Print and shaded views of the part. All mm, measured from the part's lowest x, y and z. A direction names the side the tool comes from. Coordinates: 2 decimals unless noted, no trailing zeros. Order: outer loops, then holes, each group sorted by start corner. A loop starts at its lowest first (then second) coordinate and runs counter-clockwise, first axis right, second up. Notation, with made-up numbers: M 34.25,73.5 L 60.25,73.5 A20 cw 60.25,94.5 Z; hole C 70,2 d8. An arc over 180 degrees is marked long. One line per item, written item: value.
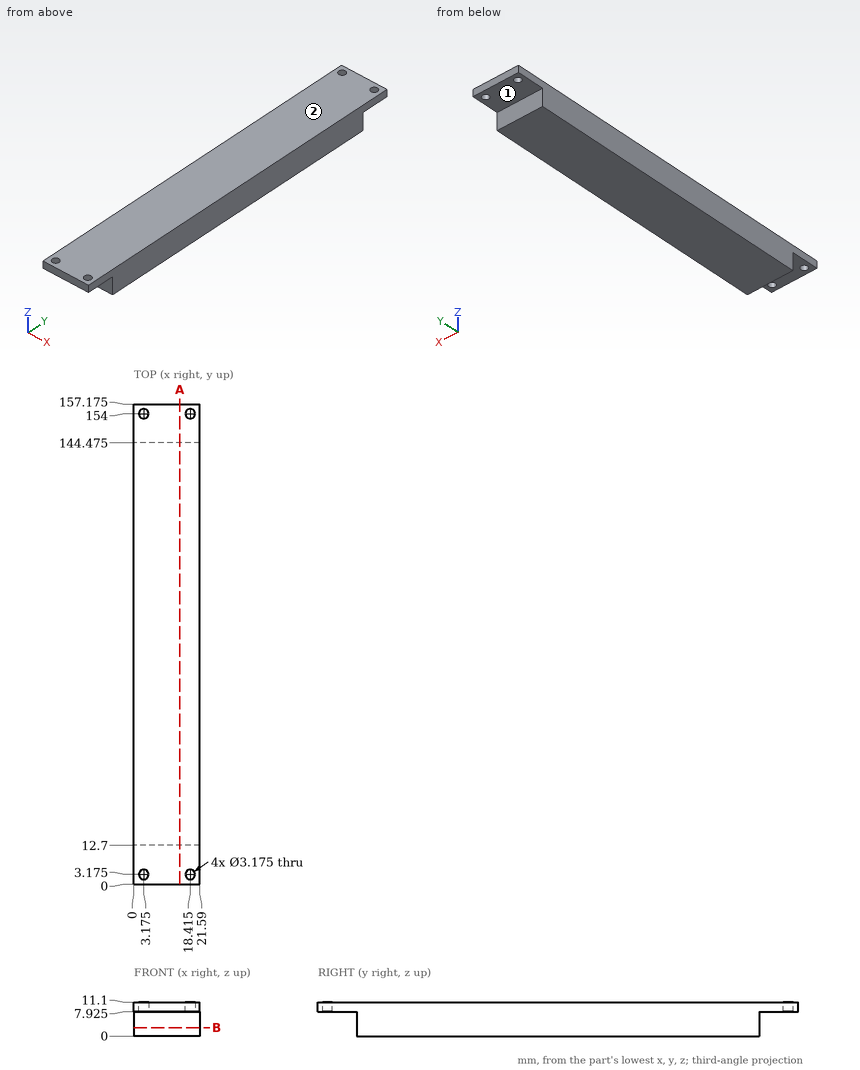
Q1. Drill centre lines: line 1 along Y through (x, z) = (3.5, 7.75) (1 decimal); line 2 along Z through (x, y) = (2.75, 8) (1 decimal). Where is each one in solid material? Low to high.
Recorded:
line 1: y = 12.7 to 144.5
line 2: z = 7.9 to 11.1
Q2. Slice it at A-A (x = 15). List the corners of the cut face in (y, z) (1 decimal), plus the area to 3 significant figures.
Recorded:
outline: M 0,7.9 L 12.7,7.9 L 12.7,0 L 144.5,0 L 144.5,7.9 L 157.2,7.9 L 157.2,11.1 L 0,11.1 Z
area: 1,540 mm^2
Q3. Pin check, flat tips, straight feed: pin 1 Ø4 at (x, y) = (3.175, 3.175) entering from -Z (3 decimals); pin 2 Ø4 at (x, z) = (8.5, 3) entering from -Y; pin 3 Ø2.5 at (x, z) = (14, 4.5) entering from +Y (3 decimals). Stop position of each tip, or through.
Recorded:
pin 1: stops at z = 7.925
pin 2: stops at y = 12.7
pin 3: stops at y = 144.475
Q4. Which spindle directions (+Z, -Z, +X, -X, +Y, -Y) get a long thin tool onto all of the face, cutting with end or side? Do the marked faces 1 and 2. Say none if no direction does.
Recorded:
face 1: -Z, +X, -X, +Y
face 2: +Z, +X, -X, +Y, -Y
Q5. Slice it at B-B (z = 2.75). List the corners of the cut face in (x, y) (1 decimal).
Recorded:
outline: M 0,12.7 L 21.6,12.7 L 21.6,144.5 L 0,144.5 Z
